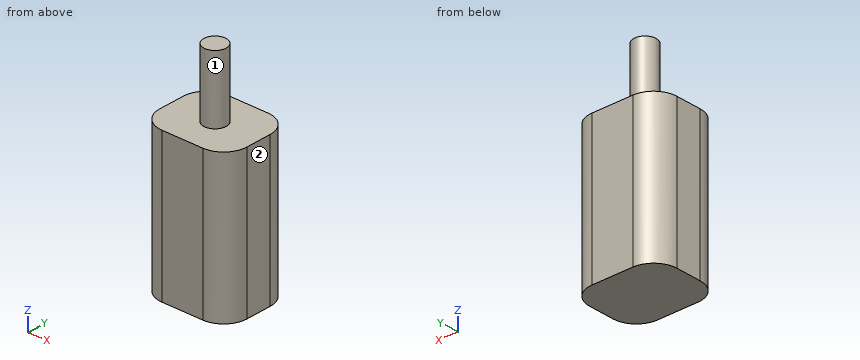
Autodesk Inventor part; units mm, degrees
ref_plane "YZ Plane" through (0, 0, 0) normal (1, 0, 0) x (0, 1, 0)
ref_plane "XZ Plane" through (0, 0, 0) normal (0, 1, 0) x (-1, 0, 0)
ref_plane "XY Plane" through (0, 0, 0) normal (0, 0, 1) x (1, 0, 0)
sketch "Sketch1" plane through (0, 0, 0) normal (0, 0, 1) x (1, 0, 0)
  line L0 (0, 0) -> (11.938, 0)
  line L1 (11.938, 0) -> (11.938, 9.906)
  line L2 (11.938, 9.906) -> (0, 9.906)
  line L3 (0, 9.906) -> (0, 0)
  circle A0 centre (5.969, 4.953) radius 1.524
  point P0 (0, 4.953)
  point P1 (5.969, 9.906)
  dimension "d0" = 11.938
  dimension "d1" = 9.906
  dimension "d2" = 3.048
extrude "Extrusion1" add sketch "Sketch1" along normal blind 20.066 contours L3 L2 L1 L0 | A0
extrude "Extrusion2" add sketch "Sketch1" along normal blind 29.21 contours A0
fillet "Fillet1" radius 3.175 4 edges at (11.938, 9.906, 10.033) (11.938, 0, 10.033) (0, 9.906, 10.033) (0, 0, 10.033)
properties part number "OGGearMotor" material "Steel, Carbon"
Geometry: final body of the model. Coordinates: model frame, mm. Face numbers are marked on the shaded views. A direction names the side the tool comes from. Round coordinates to 2 decimals unless told otherwise and drop trailing zeros. Order: outer loops, then holes, each group sorted by start corner. A loop starts at its lowest first (then second) coordinate and runs counter-clockwise, first axis right, second up. Notation, with made-up numbers: M 82.25,18.25 L 99.25,18.25 A22 cw 99.25,57.25 Z; hole C -15,39 d1. An arc over 180 degrees is marked long. Use one line per item in the form item = value. Start each with the question number.
Q1. Cut plane B-B (y = 5.25). Return loops of the section in (x, z).
Q2. Material intervals for line 1 (Z direction, x = 10, y = 6.25); line 2 (Y direction, x = 3, z = 8); line 3 (X direction, y = 7.25, z = 15.25), sorted ascending. Write a range as [from, to].
Q3. Cut plane D-D (x = 2.5). Return loops of the section in (y, z).
Q4. Cut plane A-A (z = 10.25). Return loops of the section in (x, y) (3 decimals).
Q5. Access query for the marked faces 1 and 2. Directions: +Z, -Z, +X, -X, +Y, -Y. A direction counts if a zero-diameter tool reaches every point of the face in a straight line with its end or side. Return the directions, or none.
Q6. Pin query (flat end, axial travel): pin 1 Ø5 at (x, y) = (3.5, 6.5) entering from +Z; pin 2 Ø1 at (y, z) = (2.5, 4.5) entering from +X; pin 3 Ø1.5 at (y, z) = (2, 26) entering from +X; pin 4 Ø3 at (x, z) = (8, 25.5) entering from +Y. Return the tip coordinate at first contact, or that it passes through.
Q7. Cut plane C-C (x = 1). Return loops of the section in (y, z), and give its area (3 significant figures).
Geometry results:
q1.outline = M 0,0 L 11.94,0 L 11.94,20.07 L 7.46,20.07 L 7.46,29.21 L 4.47,29.21 L 4.47,20.07 L 0,20.07 Z
q2.line_1 = [0, 20.07]
q2.line_2 = [0, 9.9]
q2.line_3 = [0.04, 11.9]
q3.outline = M 0.07,0 L 9.83,0 L 9.83,20.07 L 0.07,20.07 Z
q4.outline = M 0,3.175 A3.175 ccw 3.175,0 L 8.763,0 A3.175 ccw 11.938,3.175 L 11.938,6.731 A3.175 ccw 8.763,9.906 L 3.175,9.906 A3.175 ccw 0,6.731 Z
q5.face_1 = +Z
q5.face_2 = +Z, -Z, +X, +Y, -Y
q6.pin_1 = 29.21
q6.pin_2 = 11.93
q6.pin_3 = through
q6.pin_4 = 6.38
q7.outline = M 0.86,0 L 9.04,0 L 9.04,20.07 L 0.86,20.07 Z
q7.area = 164 mm^2
